The listing builds one solid part. Answer for the finished solid, in the listing's coordinates (mm). A direction names the side the tool comes from. Give positions to 0.01 mm unless a question says otherwise; leave off trailing zeros. Order: outer loops, then holes, each group sorted by start corner. A loop starts at its lowest first (then second) coordinate and runs counter-clockwise, first axis right, second up. Notation, with made-up numbers: (38, 63.5) -> (43, 63.5) arc R22 cw to (43, 69.5) -> close; hole circle Ø9 at (-12, 30.5). An arc over 180 degrees is marked (long way). One line per question, with ' | ' between items. Start each with the question number.
```python
from build123d import *

# Parameters (mm, degrees)
SKETCH1_W           = 116
SKETCH1_H           = 55
BOSS_EXTRUDE1_DEPTH = 187
SKETCH2_R           = 27.163974649
BOSS_EXTRUDE2_DEPTH = 17
CIRPATTERN1_COUNT   = 4
CIRPATTERN1_ANGLE   = 60


with BuildPart() as part:
    # Sketch1 → Boss-Extrude1 (new body)
    with BuildSketch(Plane(origin=(0, 0, 0), x_dir=(1, 0, 0), z_dir=(0, 1, 0))):
        Rectangle(SKETCH1_W, SKETCH1_H)
    extrude(amount=BOSS_EXTRUDE1_DEPTH)

    # Sketch2 → Boss-Extrude2 (add)
    with BuildSketch(Plane(origin=(0, 187, 0), x_dir=(1, 0, 0), z_dir=(0, 1, 0))):
        Circle(SKETCH2_R)
    extrude(amount=BOSS_EXTRUDE2_DEPTH)

    # Sketch4 → Cut-Revolve1 (revolve, cut)
    with BuildSketch(Plane(origin=(0, 194, 0), x_dir=(-1, 0, 0), z_dir=(0, 1, 0))):
        Polygon((-14.582777308, 25.258111213), (-12.417713798, 26.508111213), (-9.861835709, 22.081200504), (-12.026899219, 20.831200504), align=None)
    cut_revolve1 = revolve(axis=Axis((0, 194, 0), (0.5, 0, 0.866025404)), mode=Mode.SUBTRACT)

    # CirPattern1: Cut-Revolve1 ×4 about axis
    cirpattern1_axis = Axis((0, 0, 0), (0, -1, 0))
    for i in range(1, CIRPATTERN1_COUNT):
        add(cut_revolve1.rotate(cirpattern1_axis, i * CIRPATTERN1_ANGLE / (CIRPATTERN1_COUNT - 1)), mode=Mode.SUBTRACT)


solid = part.part
```
(1) Determine the mould class of faces 4 (the face through (-1, 92, 27.5)), 5 (the face through (-12.33, 196.44, 22.43)), 6 (the face through (-1, 0, 0)) for opening direction Z: pulls with the +Z half, pulls with the -Z half, needs draft (parallel to the pull), parting line crosses it, or undercut.
(2) The part is cut by section A-A on z = 0. Determine the outline of the cut face in (x, y).
(3) For faces 1 (the face through (58, 92, 0)), 2 (the face through (-4.1, 194, 23.7)), 3 (the face through (-27, 187, -6)), determine the directions among +Z, -Z, +X, -X, +Y, -Y from which every point of the face is accessible in a straight line to the end or side of a thin tool.
(4) Given P1, Ø10, axis at x = -11.5, z = 21.5, coming from the -Y side, flat-ended and moving along its own axis, determine where the tip first touches the part or whether it passes through.
(5) Consider line 1 (Y direction, x = -50, z = -15); line 2 (Z direction, x = 12, y = 191). Determine where each line is inside the solid, lowest interval first.
(6) The part is cut by section B-B on x = 22.5. Determine the outline of the cut face in (y, z).
(7) The part is cut by section C-C on x = 37. Determine the outline of the cut face in (y, z).
Result sheet:
1) face 4: pulls with the +Z half | face 5: undercut | face 6: needs draft
2) outline: (-58, 0) -> (58, 0) -> (58, 187) -> (27.16, 187) -> (27.16, 204) -> (-27.16, 204) -> (-27.16, 187) -> (-58, 187) -> close
3) face 1: +Z, -Z, +X, +Y, -Y | face 2: none | face 3: +Y
4) P1: stops at y = 0
5) line 1: y = 0 to 187 | line 2: z = -24.37 to 24.37
6) outline: (0, -27.5) -> (187, -27.5) -> (187, -15.22) -> (204, -15.22) -> (204, 15.22) -> (187, 15.22) -> (187, 27.5) -> (0, 27.5) -> close
7) outline: (0, -27.5) -> (187, -27.5) -> (187, 27.5) -> (0, 27.5) -> close
